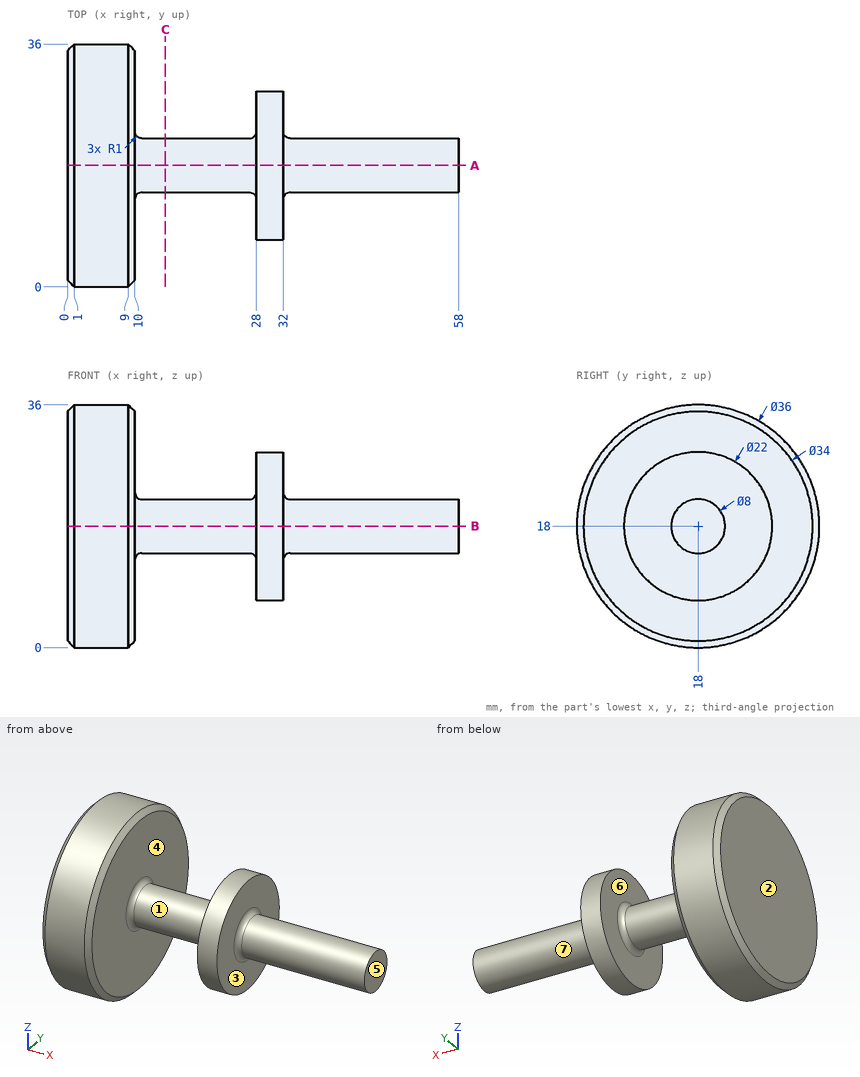
Part print with two shaded views. Sizes in mm from the minimum x, y, z corner. A direction names the side the tool comes from. Coordinates: 2 decimals unless noted, no trailing zeros. Write each loop counter-clockwise with the first axis right and the second up, starting at its lowest first coordinate (ties: lowest second). Pieces come first, ordered by that corner, then holes. Notation, with made-up numbers: (69.5, -12) - (90.5, -12) arc R19 cw to (90.5, 21) - close; hole circle Ø10 at (-0.5, 43.5). An arc over 180 degrees is marked (long way). Use a Markdown table: item, result. Add a question column.
Item 1: Band-saw the part on C-C, the plane x = 14.5. Write the cut outline in (y, z).
Item 2: 3-axis set-ups, long thin cutter, end or side, ignore diameter. For the marked faces 5, 6 and 7: which of +Z, -Z, +X, -X, +Y, -Y reach the whole face in a straight line?
Item 3: Drill centre lines: line 1 along X through (y, z) = (28, 21.5); line 2 along X through (y, z) = (31, 23); line 3 along Z through (x, y) = (54.5, 17). Where is each one in solid material? Low to high.
Item 4: Two-plate mould, pull along X, no slides. Class the marked faces 1, 2, 3 and 4: pulls with the +X half, pulls with the -X half, needs draft (parallel to the pull), parting line crosses it, or undercut.
Item 5: Band-saw the part on A-A, the plane y = 18. Write the cut outline in (x, z), and give its area (3 significant figures).
Item 6: Drop flat-ended pins along their axis: pin 1 (6 mm diameter, centred on x = 44, y = 13, fed in from +Z); pin 2 (3 mm diameter, centred on x = 41, y = 21, fed in from -Z); pin 3 (11 mm diameter, centred on y = 22.5, z = 17, fed in from +X); pin 4 (2 mm diameter, centred on y = 10.5, z = 31, fed in from +X). Give the stop position or say it passes through.
A:
| question | item | result |
|---|---|---|
| 1 | outline | circle Ø8 at (18, 18) |
| 2 | face 5 | +Z, -Z, +X, +Y, -Y |
| 2 | face 6 | none |
| 2 | face 7 | +X |
| 3 | line 1 | x = 0 to 10, 28 to 32 |
| 3 | line 2 | x = 0 to 10 |
| 3 | line 3 | z = 14.13 to 21.87 |
| 4 | face 1 | undercut |
| 4 | face 2 | pulls with the -X half |
| 4 | face 3 | pulls with the +X half |
| 4 | face 4 | undercut |
| 5 | outline | (0, 1) - (1, 0) - (9, 0) - (10, 1) - (10, 13) arc R1 cw to (11, 14) - (27, 14) arc R1 cw to (28, 13) - (28, 7) - (32, 7) - (32, 13) arc R1 cw to (33, 14) - (58, 14) - (58, 22) - (33, 22) arc R1 cw to (32, 23) - (32, 29) - (28, 29) - (28, 23) arc R1 cw to (27, 22) - (11, 22) arc R1 cw to (10, 23) - (10, 35) - (9, 36) - (1, 36) - (0, 35) - close |
| 5 | area | 799 mm² |
| 6 | pin 1 | stops at z = 21.46 |
| 6 | pin 2 | stops at z = 14.29 |
| 6 | pin 3 | stops at x = 58 |
| 6 | pin 4 | stops at x = 10 |
